Design review of the part built by this model. Coordinates are the model's own, in mm. A direction names the side the tool comes from. Round coordinates to 2 decimals unless told otherwise and drop trailing zeros. Order: outer loops, then holes, each group sorted by start corner. A loop starts at its lowest first (then second) coordinate and runs counter-clockwise, first axis right, second up. Notation, with made-up numbers: M 22,29.25 L 32,29.25 A21 cw 32,42.25 Z; hole C 9.5,89.25 d10. An arc over 180 degrees is marked long. Write item = value, one per line. Start each with the question number.
```python
from build123d import *

# Parameters (mm, degrees)
SKETCH_2_W          = 124
SKETCH_2_H          = 120
EXTRUDE_1_DEPTH     = 2
SKETCH_3_W          = 2
SKETCH_3_H          = 120
EXTRUDE_2_DEPTH     = 40
SKETCH_4_W          = 120
SKETCH_4_H          = 2
EXTRUDE_3_DEPTH     = 5
SKETCH_6_W          = 124
SKETCH_6_H          = 120
EXTRUDE_4_DEPTH     = 2.5
SKETCH_9_W          = 124
SKETCH_9_H          = 1.5
EXTRUDE_5_DEPTH     = 25
SKETCH_10_R         = 1.5
CUT_EXTRUDE_2_DEPTH = 1.5
SKETCH_11_R         = 1.5
CUT_EXTRUDE_3_DEPTH = 51
SKETCH_12_W         = 2.5
SKETCH_12_H         = 120
EXTRUDE_6_DEPTH     = 47.5
SKETCH_14_W         = 2.5
SKETCH_14_H         = 2.5
EXTRUDE_8_DEPTH     = 120
SKETCH_15_W         = 119
SKETCH_15_H         = 3
EXTRUDE_9_DEPTH     = 47.5
SKETCH_16_R         = 2.5
CUT_EXTRUDE_4_DEPTH = 10
SKETCH_18_W         = 2.5
SKETCH_18_H         = 2.5
EXTRUDE_10_DEPTH    = 120
SKETCH_20_W         = 124
SKETCH_20_H         = 25
CUT_EXTRUDE_5_DEPTH = 10
SKETCH_19_R         = 1.5
CUT_EXTRUDE_6_DEPTH = 2.5


with BuildPart() as part:
    # 草图2 → 凸台-拉伸1 (new body)
    with BuildSketch(Plane(origin=(0, 0, 0), x_dir=(1, 0, 0), z_dir=(0, 1, 0))):
        Rectangle(SKETCH_2_W, SKETCH_2_H)
    extrude(amount=EXTRUDE_1_DEPTH)

    # 草图3 → 凸台-拉伸2 (add)
    with BuildSketch(Plane(origin=(0, 2, 0), x_dir=(1, 0, 0), z_dir=(0, 1, 0))):
        with Locations((-61, 0)):
            Rectangle(SKETCH_3_W, SKETCH_3_H)
        with Locations((61, 0)):
            Rectangle(SKETCH_3_W, SKETCH_3_H)
    extrude(amount=EXTRUDE_2_DEPTH)

    # 草图4 → 凸台-拉伸3 (add)
    with BuildSketch(Plane(origin=(0, 2, 0), x_dir=(1, 0, 0), z_dir=(0, 1, 0))):
        with Locations((0, 59)):
            Rectangle(SKETCH_4_W, SKETCH_4_H)
    extrude(amount=EXTRUDE_3_DEPTH)

    # 草图6 → 凸台-拉伸4 (add)
    with BuildSketch(Plane(origin=(0, 42, 0), x_dir=(1, 0, 0), z_dir=(0, 1, 0))):
        Rectangle(SKETCH_6_W, SKETCH_6_H)
    extrude(amount=EXTRUDE_4_DEPTH)

    # 草图9 → 凸台-拉伸5 (add)
    with BuildSketch(Plane(origin=(0, 44.5, 0), x_dir=(1, 0, 0), z_dir=(0, 1, 0))):
        with Locations((0, 34.25)):
            Rectangle(SKETCH_9_W, SKETCH_9_H)
    extrude(amount=EXTRUDE_5_DEPTH)

    # 草图10 → 切除-拉伸2 (cut)
    with BuildSketch(Plane(origin=(0, 0, -35), x_dir=(-1, 0, 0), z_dir=(0, 0, -1))):
        with Locations((-22.5, 58)):
            Circle(SKETCH_10_R)
        with Locations((22.5, 58)):
            Circle(SKETCH_10_R)
    extrude(amount=-CUT_EXTRUDE_2_DEPTH, mode=Mode.SUBTRACT)

    # 草图11 → 切除-拉伸3 (cut)
    with BuildSketch(Plane(origin=(0, 44.5, 0), x_dir=(1, 0, 0), z_dir=(0, 1, 0))):
        with Locations(Location((-19.5, 1, 0), (0, 0, 270))):
            Circle(SKETCH_11_R)
        with Locations(Location((-18, 24, 0), (0, 0, 270))):
            Circle(SKETCH_11_R)
        with Locations(Location((-18, -24, 0), (0, 0, 270))):
            Circle(SKETCH_11_R)
        with Locations(Location((18, -24, 0), (0, 0, 270))):
            Circle(SKETCH_11_R)
        with Locations(Location((19.5, 1, 0), (0, 0, 270))):
            Circle(SKETCH_11_R)
        with Locations(Location((18, 24, 0), (0, 0, 270))):
            Circle(SKETCH_11_R)
    extrude(amount=-CUT_EXTRUDE_3_DEPTH, mode=Mode.SUBTRACT)

    # 草图12 → 凸台-拉伸6 (add)
    with BuildSketch(Plane.XZ):
        with Locations((-60.75, 0)):
            Rectangle(SKETCH_12_W, SKETCH_12_H)
        with Locations((60.75, 0)):
            Rectangle(SKETCH_12_W, SKETCH_12_H)
    extrude(amount=EXTRUDE_6_DEPTH)

    # 草图14 → 凸台-拉伸8 (add)
    with BuildSketch(Plane(origin=(0, 0, -60), x_dir=(-1, 0, 0), z_dir=(0, 0, -1))):
        with Locations((-58.25, -46.25)):
            Rectangle(SKETCH_14_W, SKETCH_14_H)
        with Locations((58.25, -46.25)):
            Rectangle(SKETCH_14_W, SKETCH_14_H)
    extrude(amount=-EXTRUDE_8_DEPTH)

    # 草图15 → 凸台-拉伸9 (add)
    with BuildSketch(Plane.XZ):
        with Locations((0, -58.5)):
            Rectangle(SKETCH_15_W, SKETCH_15_H)
    extrude(amount=EXTRUDE_9_DEPTH)

    # 草图16 → 切除-拉伸4 (cut)
    with BuildSketch(Plane.ZY.offset(62)):
        with Locations((2.778789214, 31.36631919)):
            Circle(SKETCH_16_R)
        with Locations((2.778789214, -33.63368081)):
            Circle(SKETCH_16_R)
    extrude(amount=-CUT_EXTRUDE_4_DEPTH, mode=Mode.SUBTRACT)

    # 草图18 → 凸台-拉伸10 (add)
    with BuildSketch(Plane.XY.offset(60)):
        with Locations((-58.25, -41.1)):
            Rectangle(SKETCH_18_W, SKETCH_18_H)
        with Locations((58.25, -41.1)):
            Rectangle(SKETCH_18_W, SKETCH_18_H)
    extrude(amount=-EXTRUDE_10_DEPTH)

    # 草图20 → 切除-拉伸5 (cut)
    with BuildSketch(Plane(origin=(0, 0, -35), x_dir=(-1, 0, 0), z_dir=(0, 0, -1))):
        with Locations((0, 57)):
            Rectangle(SKETCH_20_W, SKETCH_20_H)
    extrude(amount=-CUT_EXTRUDE_5_DEPTH, mode=Mode.SUBTRACT)

    # 草图19 → 切除-拉伸6 (cut)
    with BuildSketch(Plane(origin=(0, 44.5, 0), x_dir=(1, 0, 0), z_dir=(0, 1, 0))):
        with Locations(Location((-34.75, -29.25, 0), (0, 0, 270))):
            Circle(SKETCH_19_R)
        with Locations(Location((-34.740182935, 31.25, 0), (0, 0, 270))):
            Circle(SKETCH_19_R)
        with Locations(Location((34.75, 31.25, 0), (0, 0, 270))):
            Circle(SKETCH_19_R)
        with Locations(Location((34.75, -29.25, 0), (0, 0, 270))):
            Circle(SKETCH_19_R)
    extrude(amount=-CUT_EXTRUDE_6_DEPTH, mode=Mode.SUBTRACT)


solid = part.part
```
(1) For faces 4 (the face through (-35.653, 43.268, -32.44)), 5 (the face through (-61.01, 29.85, 0.79)), 6 (the face through (-1, 2, 0)), list the 3-axis set-ups (+Z, -Z, +X, -X, +Y, -Y) from which the entire face can be reached by the end or side of a thin tool; tool diameter is ignored.
(2) Insertion check: pin 1 (5.5 mm diameter, centred on x = 15, y = 4, fed in from +Z); pin 2 (2.5 mm diameter, centred on x = 18, z = 24, fed in from -Y); pin 3 (6 mm diameter, centred on x = -43, z = 13, fed in from -Y). Each pin has a flat end and moves straight along its axis. Give the tip position at first contact, or say it passes through.
(3) Consider section C-C, the plane y = 13.5. Write out the cut boundary in (x, z), then the cut area to 3 significant figures.
(4) Consider section D-D, the plane y = -8.5. Write out the cut boundary in (x, z), then the cut area to 3 significant figures.
(5) Consider section B-B, the plane x = -43. Write out the cut boundary in (y, z).
(6) For line 1 along Y through (x, z) = (-49.5, -24); line 2 along X through (y, z) = (-34, 14); line 3 along X through (y, z) = (-40.5, -45.5), list the stretches that pass through material, from the lowest coordinate up. Write a range as [from, to].
(7) Consider section A-A, the plane z = 38.5. Write out the cut boundary in (x, y), then the cut area to 4 significant figures.
(8) Draft analysis for pull direction Y (two halves, no side actions). For faces 1 (the face through (-0.3, -47.5, -57.5)), 2 (the face through (60, 22, 1)), 3 (the face through (-1, -21, -60)), state which applies: pulls with the +Y half, pulls with the -Y half, needs draft (parallel to the pull), parting line crosses it, or undercut.
Completed:
q1.face_4 = +Y
q1.face_5 = -X
q1.face_6 = +Z
q2.pin_1 = 60
q2.pin_2 = through
q2.pin_3 = 0
q3.outline = M -62,-60 L -60,-60 L -60,60 L -62,60 Z; M 60,-60 L 62,-60 L 62,60 L 60,60 Z
q3.area = 480 mm2
q4.outline = M -62,-60 L 62,-60 L 62,60 L 59.5,60 L 59.5,-57 L -59.5,-57 L -59.5,60 L -62,60 Z
q4.area = 957 mm2
q5.outline = M -47.5,-60 L 7,-60 L 7,-58 L 2,-58 L 2,60 L 0,60 L 0,-57 L -47.5,-57 Z; M 42,-60 L 44.5,-60 L 44.5,60 L 42,60 Z
q6.line_1 = [0, 2], [42, 44.5]
q6.line_2 = [-62, -59.5], [59.5, 62]
q6.line_3 = [-62, -57], [57, 62]
q7.outline = M -62,-47.5 L -57,-47.5 L -57,-45 L -59.5,-45 L -59.5,-42.35 L -57,-42.35 L -57,-39.85 L -59.5,-39.85 L -59.5,0 L 59.5,0 L 59.5,-39.85 L 57,-39.85 L 57,-42.35 L 59.5,-42.35 L 59.5,-45 L 57,-45 L 57,-47.5 L 62,-47.5 L 62,44.5 L -62,44.5 Z; hole M -60,2 L 60,2 L 60,42 L -60,42 Z
q7.area = 980.5 mm2
q8.face_1 = pulls with the -Y half
q8.face_2 = undercut
q8.face_3 = needs draft
